Can you work these out from the model? Positions are in its coordinate system, mm. Face numbers are marked on the shaded views. A direction names the side the tool comes from. Coordinates: 2 decimals unless noted, no trailing zeros. Write each loop counter-clockwise with the first axis right and the second up, starting at its lowest first coordinate (ties: lowest second). Pieces come first, ordered by that corner, then holes.
```python
from build123d import *

# Parameters (mm, degrees)
BOSS_EXTRUDE1_DEPTH = 15
BOSS_EXTRUDE2_DEPTH = 0.75
SKETCH6_R           = 2
CUT_EXTRUDE1_DEPTH  = 2
SKETCH7_R           = 2
CUT_EXTRUDE2_DEPTH  = 1.5


with BuildPart() as part:
    # Sketch1 → Boss-Extrude1 (new body)
    with BuildSketch(Plane.XY):
        Polygon((0, 0), (0, 10), (40, 17.053079228), (40, 2.053079228), (38, 2.053079228), (38, 14.669572043), (1.5, 8.233637247), (1.5, 0), align=None)
    extrude(amount=BOSS_EXTRUDE1_DEPTH)

    # Sketch5 → Boss-Extrude2 (add, symmetric)
    with BuildSketch(Plane(origin=(0, 0, 7.5), x_dir=(-1, 0, 0), z_dir=(0, 0, -1))):
        Polygon((-38, 14.669572043), (-38, 2.053079228), (-14.648976776, 10.552156622), align=None)
    extrude(amount=BOSS_EXTRUDE2_DEPTH, both=True)

    # Sketch6 → Cut-Extrude1 (cut)
    with BuildSketch(Plane(origin=(40, 0, 0), x_dir=(0, 0, -1), z_dir=(1, 0, 0))):
        with Locations((-4, 8.069303899)):
            Circle(SKETCH6_R)
        with Locations((-11, 8.069303899)):
            Circle(SKETCH6_R)
    extrude(amount=-CUT_EXTRUDE1_DEPTH, mode=Mode.SUBTRACT)

    # Sketch7 → Cut-Extrude2 (cut)
    with BuildSketch(Plane.ZY):
        with Locations((7.5, 5)):
            Circle(SKETCH7_R)
    extrude(amount=-CUT_EXTRUDE2_DEPTH, mode=Mode.SUBTRACT)


solid = part.part
```
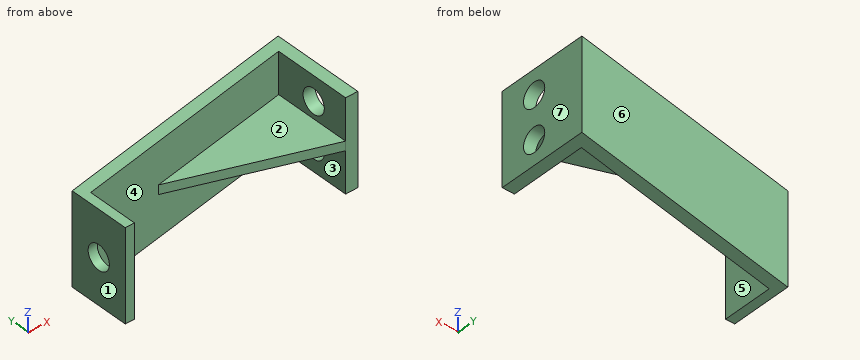
1. If we section it at C-C, the plane x = 27: List the corners of the cut face in (y, z) for me.
2. If we section it at D-D, the plane z = 1.5: List the corners of the cut face in (x, y) for me, plus the area to 3 significant figures.
3. Which directions (+Z, -Z, +X, -X, +Y, -Y) give clear straight access to the entire face, cutting with the end or side of a thin tool? Please do the marked faces 1, 2, 3 and 4.
4. If I drill on L1, parallel to X at y = 7.25, z = 1.25; L2, parallel to X at y = 1.5, z = 7.25; L3, parallel to Z at x = 29.5, y = 10.25, over which ranges is the centre line in solid material (lowest first)?
5. We'd pull the mould along X, two halves only. Please class the marked faces 5, 6 and 7: released by +X, released by -X, zero draft, split by the parting line, or undercut.
6. I'm going to push flat-ended pins straight in: P1, Ø1.5, axis at x = 28.5, y = 7.5, coming from the -Z side; P2, Ø3, axis at x = 6.5, y = 13, coming from the +Z side; P3, Ø1, axis at x = 39, z = 5, coming from the -Y side; P4, Ø4, axis at x = 11, z = 11, coming from the +Y side. Where does each tip first touch, or does it pass through?
7. If we section it at A-A, the plane z = 4: List the corners of the cut face in (x, y) for me, plus the area to 3 significant figures.
8. If we section it at B-B, the plane y = 5: List the corners of the cut face in (x, z) for me.
Answers:
1. outline: (6.06, 6.75) - (12.73, 6.75) - (12.73, 0) - (14.76, 0) - (14.76, 15) - (12.73, 15) - (12.73, 8.25) - (6.06, 8.25) - close
2. outline: (0, 0) - (1.5, 0) - (1.5, 8.23) - (38, 14.67) - (38, 2.05) - (40, 2.05) - (40, 17.05) - (0, 10) - close
2. area: 119 mm2
3. face 1: +Z, -Z, -X, +Y, -Y
3. face 2: +Z, -Y
3. face 3: -Z, -Y
3. face 4: -Y
4. L1: x = 0 to 1.5, 38 to 40
4. L2: x = 0 to 1.5
4. L3: z = 6.75 to 8.25
5. face 5: undercut
5. face 6: released by -X
5. face 7: released by +X
6. P1: stops at z = 6.75
6. P2: passes through
6. P3: stops at y = 2.05
6. P4: stops at y = 12.29
7. outline: (0, 0) - (1.5, 0) - (1.5, 8.23) - (38, 14.67) - (38, 10.07) - (40, 10.07) - (40, 17.05) - (0, 10) - close; (38, 2.05) - (40, 2.05) - (40, 6.07) - (38, 6.07) - close
7. area: 111 mm2
8. outline: (0, 0) - (1.5, 0) - (1.5, 5.5) - (0, 5.5) - close; (0, 9.5) - (1.5, 9.5) - (1.5, 15) - (0, 15) - close; (29.9, 6.75) - (38, 6.75) - (38, 0) - (40, 0) - (40, 15) - (38, 15) - (38, 8.25) - (29.9, 8.25) - close
